Geometry check sheet. Reference: the model listing, model coordinates, mm. A direction names the side the tool comes from. Give positions to 0.01 mm unless a question says otherwise; leave off trailing zeros. Order: outer loops, then holes, each group sorted by start corner. A loop starts at its lowest first (then second) coordinate and runs counter-clockwise, first axis right, second up. Notation, with made-up numbers: M 9,23 L 50,23 A14 ccw 50,42 Z; hole C 57.5,38 d9. An arc over 180 degrees is marked long. Answer as CSV lines item,"result".
from build123d import *

# Parameters (mm, degrees)
BOSS_EXTRUDE2_DEPTH = 10
SKETCH2_W           = 300
SKETCH2_H           = 5
BOSS_EXTRUDE3_DEPTH = 5
FILLET1_R           = 5
SKETCH3_W           = 380
SKETCH3_H           = 53
SKETCH3_W_2         = 80
SKETCH3_H_2         = 170
CUT_EXTRUDE1_DEPTH  = 10


with BuildPart() as part:
    # Sketch1 → Boss-Extrude2 (new body)
    with BuildSketch(Plane(origin=(0, 0, 0), x_dir=(1, 0, 0), z_dir=(0, 1, 0))):
        Polygon((-300, 105), (-250, 155), (300, 155), (300, -155), (-250, -155), (-300, -105), align=None)
    extrude(amount=BOSS_EXTRUDE2_DEPTH)

    # Sketch2 → Boss-Extrude3 (add)
    with BuildSketch(Plane(origin=(0, 10, 0), x_dir=(1, 0, 0), z_dir=(0, 1, 0))):
        with Locations((30, -87.5)):
            Rectangle(SKETCH2_W, SKETCH2_H)
        with Locations((30, 87.5)):
            Rectangle(SKETCH2_W, SKETCH2_H)
    extrude(amount=BOSS_EXTRUDE3_DEPTH)

    # Fillet1
    fillet1_edges = [part.edges().sort_by_distance(p)[0] for p in [
        (25, 0, 155),
        (-275, 0, 130),
        (-300, 0, 0),
        (-275, 0, -130),
        (25, 0, -155),
        (300, 0, 0),
    ]]
    fillet(fillet1_edges, radius=FILLET1_R)

    # Sketch3 → Cut-Extrude1 (cut)
    with BuildSketch(Plane(origin=(0, 10, 0), x_dir=(1, 0, 0), z_dir=(0, 1, 0))):
        with Locations((-10, 122.5)):
            Rectangle(SKETCH3_W, SKETCH3_H)
        with Locations((-10, -122.5)):
            Rectangle(SKETCH3_W, SKETCH3_H)
        with Locations((-150, 0)):
            Rectangle(SKETCH3_W_2, SKETCH3_H_2)
    extrude(amount=-CUT_EXTRUDE1_DEPTH, mode=Mode.SUBTRACT)


solid = part.part
(1) Gauge pin test, flat ends, axial feed: P1, Ø3, axis at y = 3, z = -15.5, coming from the -X side; P2, Ø4, axis at y = 13.5, z = -86.5, coming from the -X side; P3, Ø3, axis at x = 67, y = 3, coming from the +Z side. Record the tip position at first contact, or that the pin passes through.
The answers:
P1,"stops at x = -299.97"
P2,"stops at x = -120"
P3,"stops at z = 154.97"
(2) Section check D-D on y = 7.25. Enter the section's corners in (x, z), then the cut area to 3 significant figures.
The answers:
outline,"M -300,-105 L -250,-155 L 300,-155 L 300,155 L -250,155 L -300,105 Z; hole M -200,-149 L 180,-149 L 180,-96 L -200,-96 Z; hole M -200,96 L 180,96 L 180,149 L -200,149 Z; hole M -190,-85 L -110,-85 L -110,85 L -190,85 Z"
area,"130,000 mm2"
(3) Section check C-C on z = -12. Enter the section's corners in (x, y).
The answers:
outline,"M -300,5 A5 ccw -295,0 L -190,0 L -190,10 L -300,10 Z; M -110,0 L 295,0 A5 ccw 300,5 L 300,10 L -110,10 Z"
(4) Material ranges on line 1 (Z direction, x = 156, y = 6.5); line 2 (Z direction, x = -53.5, y = 10.25); line 3 (X direction, y = 8.25, z = 17), recorded low to high.
The answers:
line 1,"z = -155 to -149, -96 to 96, 149 to 155"
line 2,"z = -90 to -85, 85 to 90"
line 3,"x = -300 to -190, -110 to 300"
(5) Draft check along X on faces 1 (the face through (4, 0, -2)), 2 (the face through (-49, 11, -85)), 3 (the face through (-275, 7, 130)). Enter one of: +X half, -X half, draft (parallel to the pull), parting line (faces both ways), or undercut.
The answers:
face 1,"draft"
face 2,"undercut"
face 3,"-X half"
(6) Tool access check on faces 4 (the face through (-49, 11, 85)), 5 (the face through (-274.29, 1.43, 128.59)). Record the directions out of +Z, -Z, +X, -X, +Y, -Y that give a thin tool (end or side, any length) a straight path to the whole face; none if there is none.
The answers:
face 4,"+Y"
face 5,"+Z, -X, -Y"
(7) Section check B-B on x = -28.5. Enter the section's corners in (y, z).
The answers:
outline,"M 0,-150 A5 ccw 5,-155 L 10,-155 L 10,-149 L 0,-149 Z; M 0,-96 L 10,-96 L 10,-90 L 15,-90 L 15,-85 L 10,-85 L 10,85 L 15,85 L 15,90 L 10,90 L 10,96 L 0,96 Z; M 0,149 L 10,149 L 10,155 L 5,155 A5 ccw 0,150 Z"
(8) Section check A-A on x = -184. Enter the section's corners in (y, z).
The answers:
outline,"M 0,-150 A5 ccw 5,-155 L 10,-155 L 10,-149 L 0,-149 Z; M 0,-96 L 10,-96 L 10,-85 L 0,-85 Z; M 0,85 L 10,85 L 10,96 L 0,96 Z; M 0,149 L 10,149 L 10,155 L 5,155 A5 ccw 0,150 Z"
